Drawing for the job (mm, zero at the part's lowest x, y, z). A direction names the side the tool comes from. Coordinates: 2 decimals unless noted, no trailing zeros. Write each loop counter-clockwise with the first axis right and the second up, starting at its lowest first coordinate (ties: lowest second). Pieces come first, ordered by that corner, then holes. Notation, with made-up numbers: M 74.25,72.25 L 86.25,72.25 A19 ccw 86.25,102.25 Z; hole C 82.25,-25.5 d7. An arc over 180 degrees is marked long. Put each result on its own line as item: value. Start each with the question number.
Q1. Cut at C-C (z = 33.5). Write the cut outline in (x, y).
Q2. Which spindle directions (+Z, -Z, +X, -X, +Y, -Y) get a long thin tool onto all of the face, cutting with end or side? Do the marked faces 1 and 2. Say none if no direction does.
Q3. Drop a flat-ended pin along its axis: pin 1 (4.5 mm diameter, centred on x = 26.5, y = 3, fed in from -Z). Give the stop position or say it passes through.
Q4. Drill centre lines: line 1 along Z through (x, y) = (22.5, 4.5); line 2 along Z through (x, y) = (30.5, 4.75); line 3 along X through (y, z) = (3.75, 14). Where is each one in solid material? Low to high.
Q5. Pull direction X, two halves, no side cores. Call the marked faces 3, 4, 5 and 6: pulls with the +X half, pulls with the -X half, needs draft (parallel to the pull), parting line crosses it, or undercut.
Q6. Cut at B-B (y = 1.75). Write the cut outline in (x, z), then the cut area to 3 significant figures.
Q7. Cut at A-A (x = 11.5). Write the cut outline in (y, z), then the cut area to 3 significant figures.
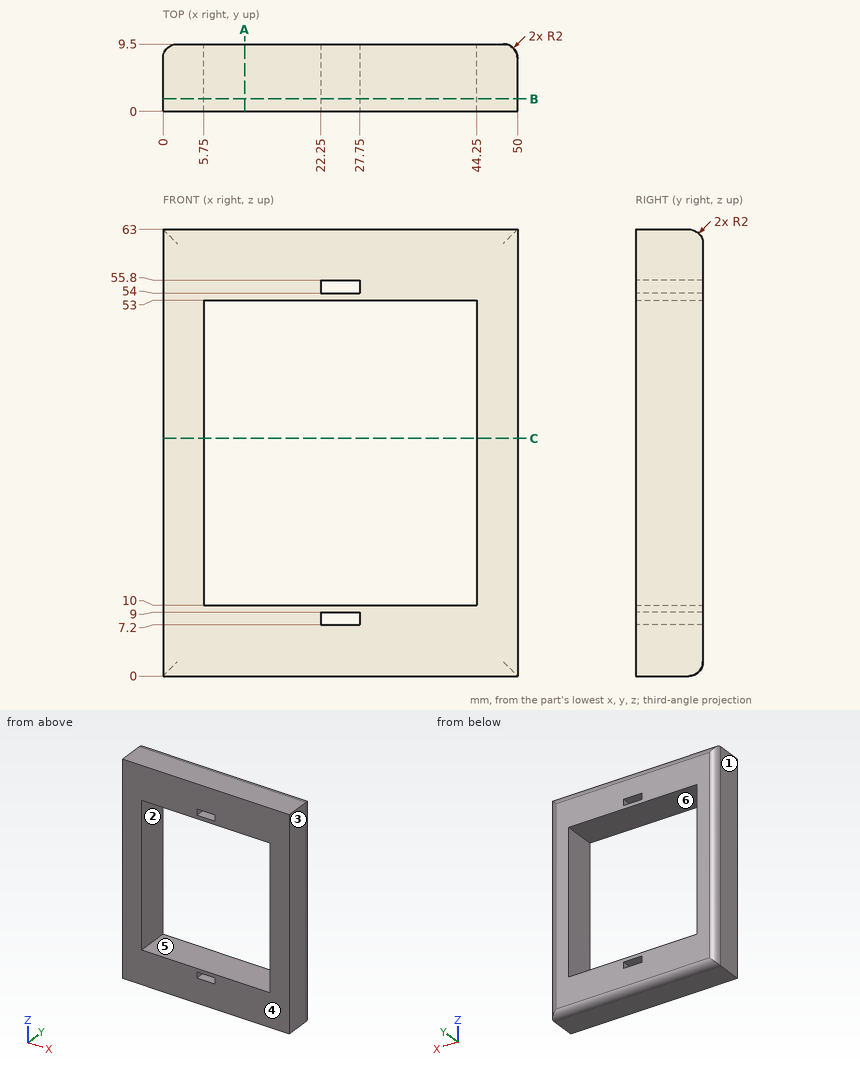
Computed values:
1. outline: M 0,0 L 5.75,0 L 5.75,9.5 L 2,9.5 A2 ccw 0,7.5 Z; M 44.25,0 L 50,0 L 50,7.5 A2 ccw 48,9.5 L 44.25,9.5 Z
2. face 1: +Z, -Z, -X, +Y, -Y
2. face 2: +Y, -Y
3. pin 1: z = 0
4. line 1: 0 to 7.2, 9 to 10, 53 to 54, 55.8 to 63
4. line 2: 0 to 10, 53 to 63
4. line 3: 0 to 5.75, 44.25 to 50
5. face 3: pulls with the +X half
5. face 4: needs draft
5. face 5: undercut
5. face 6: undercut
6. outline: M 0,0 L 50,0 L 50,63 L 0,63 Z; hole M 5.75,10 L 44.25,10 L 44.25,53 L 5.75,53 Z; hole M 22.25,7.2 L 27.75,7.2 L 27.75,9 L 22.25,9 Z; hole M 22.25,54 L 27.75,54 L 27.75,55.8 L 22.25,55.8 Z
6. area: 1,470 mm2
7. outline: M 0,0 L 7.5,0 A2 ccw 9.5,2 L 9.5,10 L 0,10 Z; M 0,53 L 9.5,53 L 9.5,61 A2 ccw 7.5,63 L 0,63 Z
7. area: 188 mm2
